Source: CAD feature listing. Evaluate the final solid. Frame: model axes, mm. A direction names the side the tool comes from. Coordinates: 2 decimals unless noted, no trailing zeros. Loops run counter-clockwise (first coordinate to the right, second up) from the corner with the lowest first, then second, coordinate; pieces in that order, holes last.
Item 1: Section query A-A, the plane z = 3.9. Return the cut outline in (x, y).
Item 2: Section query C-C, the plane y = 15.5. Return the cut outline in (x, z).
Item 3: Pull-direction query (Y, two-part tool) for faces 1 (the flat face through (66.042, 3, 2)), 2 (the flat face through (-1, 41.413, 2)), 3 (the flat face through (62.982, 3, 3)), 4 (the flat face through (-63.818, 3, 3)); classes: +Y half, -Y half, draft (parallel to the pull), parting line (faces both ways), or undercut.
Item 4: Reachability of faces 5 (the flat face through (-1, -31.367, 3)), 6 (the flat face through (-66.878, 3, 2)) from +Z, -Z, +X, -X, +Y, -Y: full face, straight path, thin tool, end or side. Return the list, or none.
Item 5: Pin query (flat end, axial travel): pin 1 Ø1.1 at (y, z) = (16, 5.5) entering from +X; pin 2 Ø23 at (x, y) = (1.5, 7) entering from +Z; pin 3 Ø0.5 at (y, z) = (-11.5, 5.5) entering from -X. Return the tip coordinate at first contact, or that it passes through.
Item 6: Line query: probe 1 along Y at (x, z) = (-21.5, 4); probe 2 along X at (y, z) = (-15.5, 2.45); probe 3 along Y at (x, z) = (-49.5, 5.2). Output: solid intervals per line, ascending.
Item 7: Section query B-B, the plane x = 24.5. Return the cut outline in (y, z).
```python
from build123d import *

# Parameters (mm, degrees)
F0_W     = 128.72
F0_H     = 71.64
F0_W_2   = 126.8
F0_H_2   = 69.72
F1_DEPTH = 6
F0_W_3   = 132.92
F0_H_3   = 75.84
F2_DEPTH = 5
F3_DEPTH = 1
F5_SIZE  = 1
F6_SIZE  = 2


with BuildPart() as f1:
    # F0 (on Top) → F1 (new body)
    with BuildSketch(Plane.XY):
        with Locations((9.5820501447, 3.493278903)):
            Rectangle(F0_W, F0_H)
        with Locations((9.5820501447, 3.493278903)):
            Rectangle(F0_W_2, F0_H_2, mode=Mode.SUBTRACT)
    extrude(amount=F1_DEPTH)

    # F0 (on Top) → F2 (join)
    with BuildSketch(Plane.XY):
        with Locations((9.5820501447, 3.493278903)):
            Rectangle(F0_W_3, F0_H_3)
        with Locations((9.5820501447, 3.493278903)):
            Rectangle(F0_W, F0_H, mode=Mode.SUBTRACT)
    extrude(amount=F2_DEPTH)

    # F0 (on Top) → F3 (join)
    with BuildSketch(Plane.XY):
        with Locations((9.5820501447, 3.493278903)):
            Rectangle(F0_W_2, F0_H_2)
    extrude(amount=F3_DEPTH)


with BuildPart() as f1_1:
    # F4: moved
    add(f1.part.moved(Location((-10, 0, 0))))

    # F5
    f5_edges = [f1_1.edges().sort_by_distance(p)[0] for p in [
        (-64.77795, -32.326721, 5.5),
        (63.94205, -32.326721, 5.5),
        (63.94205, 39.313279, 5.5),
        (-64.77795, 39.313279, 5.5),
    ]]
    chamfer(f5_edges, length=F5_SIZE)

    # F6
    f6_edges = [f1_1.edges().sort_by_distance(p)[0] for p in [
        (-66.87795, 41.413279, 2.5),
        (-66.87795, -34.426721, 2.5),
        (66.04205, -34.426721, 2.5),
        (66.04205, 41.413279, 2.5),
    ]]
    chamfer(f6_edges, length=F6_SIZE)


solid = f1_1.part
```
Verdict:
1. outline: (-66.88, -32.43) - (-64.88, -34.43) - (64.04, -34.43) - (66.04, -32.43) - (66.04, 39.41) - (64.04, 41.41) - (-64.88, 41.41) - (-66.88, 39.41) - close; hole (-63.82, -31.37) - (62.98, -31.37) - (62.98, 38.35) - (-63.82, 38.35) - close
2. outline: (-66.88, 0) - (66.04, 0) - (66.04, 5) - (63.94, 5) - (63.94, 6) - (62.98, 6) - (62.98, 1) - (-63.82, 1) - (-63.82, 6) - (-64.78, 6) - (-64.78, 5) - (-66.88, 5) - close
3. face 1: draft
3. face 2: +Y half
3. face 3: undercut
3. face 4: undercut
4. face 5: +Z
4. face 6: +Z, -Z, -X, +Y, -Y
5. pin 1: stops at x = 66.04
5. pin 2: stops at z = 1
5. pin 3: stops at x = -64.78
6. probe 1: y = -34.43 to -31.37, 38.35 to 41.41
6. probe 2: x = -66.88 to -63.82, 62.98 to 66.04
6. probe 3: y = -32.33 to -31.37, 38.35 to 39.31
7. outline: (-34.43, 0) - (41.41, 0) - (41.41, 5) - (39.31, 5) - (39.31, 6) - (38.35, 6) - (38.35, 1) - (-31.37, 1) - (-31.37, 6) - (-32.33, 6) - (-32.33, 5) - (-34.43, 5) - close
